Geometry check sheet. Reference: the model listing, model coordinates, mm. A direction names the side the tool comes from. Round coordinates to 2 decimals unless told otherwise and drop trailing zeros. Write each loop counter-clockwise with the first axis right and the second up, starting at its lowest first coordinate (ties: lowest second). Pieces come first, ordered by that corner, then holes. Notation, with made-up numbers: M 50,19.5 L 94,19.5 A33 cw 94,55.5 Z; hole C 19.5,70 d11. An arc over 180 degrees is marked long. Answer in a Markdown table with one row per item. Add a question column.
from build123d import *

# Parameters (mm, degrees)
F1_DEPTH = 63.5
F2_DEPTH = 12.7
F3_DEPTH = 8.0645
F5_R     = 6.35


# Not quite as in the source:
# - ends of sketch curves that miss each other by under 0.0002 mm in the source are joined


with BuildPart() as f1:
    # F0 (on Front) → F1 (new body, symmetric)
    with BuildSketch(Plane.XZ):
        Polygon((-41.275, -9.525), (41.275, -9.525), (41.275, 9.525), (22.225, 9.525), (-41.275, 9.525), align=None)
    extrude(amount=F1_DEPTH, both=True)

    # F0 (on Front) → F2 (join, symmetric)
    with BuildSketch(Plane.XZ):
        with BuildLine():
            Line((22.225, 9.525), (41.275, 9.525))
            Line((41.275, 9.525), (41.275, 27.0002))
            ThreePointArc((41.275, 27.0002), (45.9246798487, 38.2255201513), (57.15, 42.8752))
            Line((57.15, 42.8752), (60.325, 42.8752))
            Line((60.325, 42.8752), (60.325, 61.9252))
            Line((60.325, 61.9252), (57.15, 61.9252))
            ThreePointArc((57.15, 61.9252), (32.4542956671, 51.6959043329), (22.225, 27.0002))
            Line((22.225, 27.0002), (22.225, 9.525))
        make_face()
        Polygon((85.7250011283, 61.9252), (60.325, 61.9252), (60.325, 42.8752), (85.725, 42.8752), align=None)
    extrude(amount=F2_DEPTH, both=True)

    # F0 (on Front) → F3 (join, symmetric)
    with BuildSketch(Plane.XZ):
        with BuildLine():
            add(Edge.make_bspline(
                [(-41.275, 9.525), (-41.275, 36.3431351324), (6.7984250959, 61.9252), (57.15, 61.9252)],
                knots=[0, 0, 0, 0, 111.5045361635, 111.5045361635, 111.5045361635, 111.5045361635], degree=3))
            Line((-41.275, 9.525), (22.225, 9.525))
            Line((22.225, 9.525), (22.225, 27.0002))
            ThreePointArc((22.225, 27.0002), (32.4542956671, 51.6959043329), (57.15, 61.9252))
        make_face()
    extrude(amount=F3_DEPTH, both=True)

    # F0 (on Front) → F4 (revolve)
    with BuildSketch(Plane.XZ):
        Polygon((85.725, 66.675), (85.725, 61.9252), (85.725, 42.8752), (85.725, 38.1), (111.125, 38.1), (111.125, 66.675), align=None)
    revolve(axis=Axis((85.725, 0, 52.3875), (0, 0, 1)))

    # F5
    f5_edges = [f1.edges().sort_by_distance(p)[0] for p in [
        (41.275, -63.5, 0),
        (-41.275, -63.5, 0),
        (-41.275, 63.5, 0),
        (41.275, 63.5, 0),
    ]]
    fillet(f5_edges, radius=F5_R)


solid = f1.part
Item 1: Mould release check, pull along X, two halves, no side actions. Record for faces 6 (the cylindrical face through (45.8, -0.2, 38.1)), 7 (the flat face through (0, 63.5, 0)), 8 (the cylindrical face through (39.464, 61.59, 0.133)): +X half, -X half, draft (parallel to the pull), parting line (faces both ways), or undercut.
Item 2: Access from +Z, -Z, +X, -X, +Y, -Y to the whole of each face (thin tool, end or side, straight path). Record for faces 1 (the flat face through (38, 12.7, 36)), 2 (the flat face through (41.275, -1, 4)), 3 (the flat face through (60, 0, 61.925)), 4 (the cylindrical face through (32.73, -10.41, 51.97)), 5 (the flat face through (60, 0, 42.875)).
Item 3: Scan lines: probe 1 along Z at (x, y) = (26, -56.5) (3 decimals); probe 2 along Y at (x, z) = (16, 30); probe 3 along X at (y, z) = (-44, 7) (3 decimals). Record each from-to range of solid material in increasing order. Write a range as from..to.
Item 4: Gauge pin test, flat ends, axial feed: pin 1 Ø21 at (x, z) = (47.5, 46.5) entering from +Y; pin 2 Ø1 at (x, y) = (38, -50) entering from +Z (3 decimals); pin 3 Ø2 at (x, z) = (-9.5, 16) entering from +Y; pin 4 Ø5.5 at (x, y) = (60.5, -4) entering from +Z (3 decimals). Record the tip position at first contact, or that the pin passes through.
Item 5: Section check A-A, the plane y = 50. Record the boundary of the cut face in (x, z) (3 decimals).
Result sheet:
| question | item | result |
|---|---|---|
| 1 | face 6 | undercut |
| 1 | face 7 | draft |
| 1 | face 8 | +X half |
| 2 | face 1 | +Z, -X, +Y |
| 2 | face 2 | -Z, +X, +Y, -Y |
| 2 | face 3 | +Z, -X |
| 2 | face 4 | +Z, -X, -Y |
| 2 | face 5 | -Z |
| 3 | probe 1 | z = -9.525..9.525 |
| 3 | probe 2 | y = -8.06..8.06 |
| 3 | probe 3 | x = -41.275..41.275 |
| 4 | pin 1 | stops at y = 12.7 |
| 4 | pin 2 | stops at z = 9.525 |
| 4 | pin 3 | stops at y = 8.06 |
| 4 | pin 4 | stops at z = 66.675 |
| 5 | outline | M -41.275,-9.525 L 41.275,-9.525 L 41.275,9.525 L -41.275,9.525 Z |
